Geometry check sheet. Reference: the model listing, model coordinates, mm. Give positions to 0.01 mm unless a question says otherwise; leave off trailing zeros. Loops run counter-clockwise (first coordinate to the right, second up) from the corner with the lowest first, then second, coordinate; pieces in that order, holes last. Notation, with made-up numbers: (-13.75, 6.5) - (10.25, 6.5) arc R15 ccw to (10.25, 19.5) - close; hole circle Ø3 at (47, 50). An arc over 180 degrees is marked (long way). Use a Markdown table: item, result. Add a question column.
1. Cross-section at C-C on x = 21.5. Enter the section's corners in (y, z), and give its area (3 significant figures).
2. Depth check by flat-ended pin: P1, Ø1.5, axis at y = 3, z = -26, coming from the -X side; P2, Ø4.5, axis at x = 27.5, z = 0, coming from the +Y side. Enter the tip coordinate at first touch or a pass-through.
3. Material ranges on L1, parallel to Z at x = 13.5, y = 1.95; L2, parallel to Z at x = 53, y = 1.15; L3, parallel to X at y = 1.25, z = -39.5 (3 decimals), recorded low to high.
4. Draft check along Z on faces 1 (the flat face through (-0.2, 2.3, 34.5)), 2 (the flat face through (36, 2.5, 1)). Enter one of: pulls with the +Z half, pulls with the -Z half, needs draft (parallel to the pull), parting line crosses it, or undercut.
5. Cross-section at A-A on z = 23. Enter the section's corners in (x, y) (3 decimals).
6. Cross-section at B-B on z = -3.5. Enter the section's corners in (x, y) (3 decimals).
7. Cross-section at D-D on z = -36. Enter the section's corners in (x, y) (3 decimals).
from build123d import *

# Parameters (mm, degrees)
SKETCH2_W           = 29.42
SKETCH2_H           = 69
SKETCH2_W_2         = 23.42
SKETCH2_H_2         = 17.5
BOSS_EXTRUDE1_DEPTH = 2.5
SKETCH2_3_R         = 0.7
BOSS_EXTRUDE2_DEPTH = 4
SKETCH3_W           = 19.2
SKETCH3_H           = 33.6
SKETCH3_W_2         = 15.2
SKETCH3_H_2         = 29.6
BOSS_EXTRUDE3_DEPTH = 2.5
SKETCH4_W           = 105
SKETCH4_H           = 95
SKETCH4_W_2         = 20
SKETCH4_H_2         = 4
BOSS_EXTRUDE4_DEPTH = 2


with BuildPart() as part:
    # Sketch2 → Boss-Extrude1 (new body)
    with BuildSketch(Plane(origin=(0, 0, 0), x_dir=(1, 0, 0), z_dir=(0, 1, 0))):
        Rectangle(SKETCH2_W, SKETCH2_H)
        Polygon((11.71, -11), (-11.71, -11), (-11.71, 29.5), (-9.3, 29.5), (-9.3, 31.5), (9.3, 31.5), (9.3, 29.5), (11.71, 29.5), align=None, mode=Mode.SUBTRACT)
        with Locations((0, -22.75)):
            Rectangle(SKETCH2_W_2, SKETCH2_H_2, mode=Mode.SUBTRACT)
    extrude(amount=BOSS_EXTRUDE1_DEPTH)

    # Sketch2<3> → Boss-Extrude2 (add)
    with BuildSketch(Plane(origin=(0, 0, 0), x_dir=(1, 0, 0), z_dir=(0, 1, 0))):
        with Locations(Location((-10.8, 31, 0), (0, 0, 270))):
            Circle(SKETCH2_3_R)
        with Locations(Location((-5.21, -12.5, 0), (0, 0, 270))):
            Circle(SKETCH2_3_R)
        with Locations(Location((10.8, 31, 0), (0, 0, 90))):
            Circle(SKETCH2_3_R)
    extrude(amount=BOSS_EXTRUDE2_DEPTH)



with BuildPart() as body_2:
    # Sketch3 → Boss-Extrude3 (new body)
    with BuildSketch(Plane(origin=(0, 0, 0), x_dir=(1, 0, 0), z_dir=(0, 1, 0))):
        with Locations((44.31, 0)):
            Rectangle(SKETCH3_W, SKETCH3_H)
        with Locations((44.31, 0)):
            Rectangle(SKETCH3_W_2, SKETCH3_H_2, mode=Mode.SUBTRACT)
    extrude(amount=BOSS_EXTRUDE3_DEPTH)


with BuildPart() as part_1:
    add(part.part)

    add(body_2.part)  # Boss-Extrude4 merges body 2
    # Sketch4 → Boss-Extrude4 (add)
    # profile 1 of 2: a face of its own
    with BuildSketch(Plane(origin=(0, 0, 0), x_dir=(1, 0, 0), z_dir=(0, 1, 0))):
        with Locations((22.155, 0)):
            Rectangle(SKETCH4_W, SKETCH4_H)
        Polygon((-25.345, -42.5), (-25.345, -2), (-14.71, -2), (-14.71, 2), (-25.345, 2), (-25.345, 42.5), (-2, 42.5), (-2, 34.5), (2, 34.5), (2, 42.5), (42.31, 42.5), (42.31, 16.8), (46.31, 16.8), (46.31, 42.5), (69.655, 42.5), (69.655, 2), (53.91, 2), (53.91, -2), (69.655, -2), (69.655, -42.5), (46.31, -42.5), (46.31, -16.8), (42.31, -16.8), (42.31, -42.5), (2, -42.5), (2, -34.5), (-2, -34.5), (-2, -42.5), align=None, mode=Mode.SUBTRACT)
    # profile 2 of 2: a face of its own
    with BuildSketch(Plane(origin=(0, 0, 0), x_dir=(1, 0, 0), z_dir=(0, 1, 0))):
        with Locations((24.71, 0)):
            Rectangle(SKETCH4_W_2, SKETCH4_H_2)
    extrude(amount=BOSS_EXTRUDE4_DEPTH)


solid = part_1.part
Values found:
| question | item | result |
|---|---|---|
| 1 | outline | (0, -47.5) - (2, -47.5) - (2, -42.5) - (0, -42.5) - close; (0, -2) - (2, -2) - (2, 2) - (0, 2) - close; (0, 42.5) - (2, 42.5) - (2, 47.5) - (0, 47.5) - close |
| 1 | area | 28.0 mm2 |
| 2 | P1 | stops at x = -14.71 |
| 2 | P2 | stops at y = 2 |
| 3 | L1 | z = -47.5 to -42.5, -34.5 to 34.5, 42.5 to 47.5 |
| 3 | L2 | z = -47.5 to -42.5, -16.8 to 16.8, 42.5 to 47.5 |
| 3 | L3 | x = -30.345 to -25.345, -2 to 2, 42.31 to 46.31, 69.655 to 74.655 |
| 4 | face 1 | undercut |
| 4 | face 2 | needs draft |
| 5 | outline | (-30.345, 0) - (-25.345, 0) - (-25.345, 2) - (-30.345, 2) - close; (-14.71, 0) - (-11.71, 0) - (-11.71, 2.5) - (-14.71, 2.5) - close; (11.71, 0) - (14.71, 0) - (14.71, 2.5) - (11.71, 2.5) - close; (42.31, 0) - (46.31, 0) - (46.31, 2) - (42.31, 2) - close; (69.655, 0) - (74.655, 0) - (74.655, 2) - (69.655, 2) - close |
| 6 | outline | (-30.345, 0) - (-25.345, 0) - (-25.345, 2) - (-30.345, 2) - close; (-14.71, 0) - (-11.71, 0) - (-11.71, 2.5) - (-14.71, 2.5) - close; (11.71, 0) - (14.71, 0) - (14.71, 2.5) - (11.71, 2.5) - close; (34.71, 0) - (36.71, 0) - (36.71, 2.5) - (34.71, 2.5) - close; (51.91, 0) - (53.91, 0) - (53.91, 2.5) - (51.91, 2.5) - close; (69.655, 0) - (74.655, 0) - (74.655, 2) - (69.655, 2) - close |
| 7 | outline | (-30.345, 0) - (-25.345, 0) - (-25.345, 2) - (-30.345, 2) - close; (-2, 0) - (2, 0) - (2, 2) - (-2, 2) - close; (42.31, 0) - (46.31, 0) - (46.31, 2) - (42.31, 2) - close; (69.655, 0) - (74.655, 0) - (74.655, 2) - (69.655, 2) - close |
